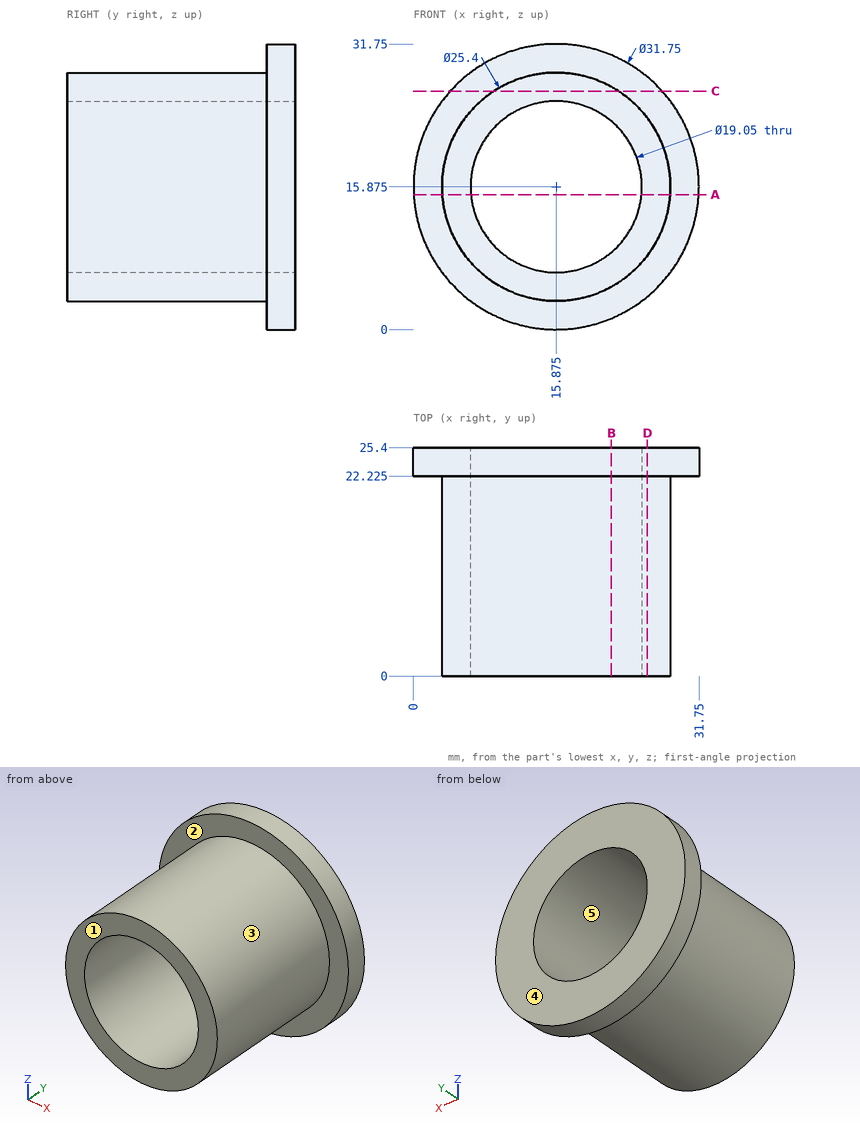
Job drawing, mm, ordinate dimensions from the low corner. One solid piece. A direction names the side the tool comes from. Coordinates: 2 decimals unless noted, no trailing zeros. Order: outer loops, then holes, each group sorted by start corner. A loop starts at its lowest first (then second) coordinate and runs counter-clockwise, first axis right, second up. Notation, with made-up numbers: (-18, 49) - (-14, 49) arc R5 ccw to (-14, 53) - close; hole circle Ø7 at (31, 0). An arc over 180 degrees is marked (long way). Write each question's results on one line, items separated by ' | '. Start each with the question number.
Item 1: Band-saw the part on A-A on z = 15. Write the cut outline in (x, y) (3 decimals).
Item 2: Tool access for the marked faces 1 and 2: list every direction of +Z, -Z, +X, -X, +Y, -Y with a clear straight run to the whole face (end or side of a thin tool).
Item 3: Flat gauge pins, fed straight in: pin 1 (4 mm diameter, centred on y = 9.5, z = 22, fed in from +X); pin 2 (1 mm diameter, centred on y = 9.5, z = 17, fed in from -X); pin 3 (10 mm diameter, centred on y = 22.5, z = 4.5, fed in from +X). Where does each tip first touch, or does it go through?
Item 4: Band-saw the part on C-C on z = 26.5. Write the cut outline in (x, y) (3 decimals).
Item 5: Wall check: probe 1 along Y at (x, z) = (26, 25) (3 decimals); probe 2 along Z at (x, y) = (15, 9); probe 3 along Z at (x, y) = (11, 21.75). Give the ranges that are in metal, low to high. Write a range as [from, to].
Item 6: Mould opens along X. For the marked faces 3, 4 and 5 say: released by +X, released by -X, zero draft, split by the parting line, or undercut.
Item 7: Band-saw the part on D-D on x = 26. Write the cut outline in (y, z) (3 decimals), and give its area (3 significant figures).
Item 8: Band-saw the part on B-B on x = 22. Write the cut outline in (y, z) (3 decimals).
Numbers:
1) outline: (0.024, 22.225) - (3.205, 22.225) - (3.205, 0) - (6.39, 0) - (6.39, 25.4) - (0.024, 25.4) - close; (25.36, 0) - (28.545, 0) - (28.545, 22.225) - (31.726, 22.225) - (31.726, 25.4) - (25.36, 25.4) - close
2) face 1: +Z, -Z, +X, -X, -Y | face 2: -Y
3) pin 1: x = 27.89 | pin 2: x = 3.19 | pin 3: x = 30.41
4) outline: (4.08, 22.225) - (8.918, 22.225) - (8.918, 0) - (22.832, 0) - (22.832, 22.225) - (27.67, 22.225) - (27.67, 25.4) - (4.08, 25.4) - close
5) probe 1: [22.225, 25.4] | probe 2: [3.21, 6.39], [25.36, 28.54] | probe 3: [4.15, 7.69], [24.06, 27.6]
6) face 3: split by the parting line | face 4: zero draft | face 5: undercut
7) outline: (0, 8.209) - (22.225, 8.209) - (22.225, 3.648) - (25.4, 3.648) - (25.4, 28.102) - (22.225, 28.102) - (22.225, 23.541) - (0, 23.541) - close | area: 418 mm^2
8) outline: (0, 4.75) - (22.225, 4.75) - (22.225, 1.229) - (25.4, 1.229) - (25.4, 8.58) - (0, 8.58) - close; (0, 23.17) - (25.4, 23.17) - (25.4, 30.521) - (22.225, 30.521) - (22.225, 27) - (0, 27) - close
